```python
from build123d import *

# Parameters (mm, degrees)
BOSS_EXTRUDE1_DEPTH     = 6.35
F_1_4_CLEARANCE_HOLE1_D = 6.7564
FILLET1_R               = 2.54
SKETCH4_R               = 3.175
CUT_EXTRUDE1_DEPTH      = 7.3500001


with BuildPart() as part:
    # Sketch1 → Boss-Extrude1 (new body)
    with BuildSketch(Plane(origin=(0, 0, 0), x_dir=(1, 0, 0), z_dir=(0, 1, 0))):
        with BuildLine():
            ThreePointArc((34.041521739, -4.120545799), (22.86, 0), (34.041521739, 4.120545799))
            ThreePointArc((34.041521739, 4.120545799), (-34.29, 0), (34.041521739, -4.120545799))
        make_face()
    extrude(amount=BOSS_EXTRUDE1_DEPTH)

    # 1/4 Clearance Hole1 (through all)
    with Locations(Plane(origin=(0, 6.35, 0), x_dir=(1, 0, 0), z_dir=(0, 1, 0))):
        with Locations((0, 0)):
            Hole(F_1_4_CLEARANCE_HOLE1_D / 2)

    # Fillet1
    fillet1_edges = [part.edges().sort_by_distance(p)[0] for p in [
        (34.041521739, 3.175, 4.120545799),
        (34.041521739, 3.175, -4.120545799),
    ]]
    fillet(fillet1_edges, radius=FILLET1_R)

    # Sketch4 → Cut-Extrude1 (cut, through all)
    with BuildSketch(Plane(origin=(0, 6.35, 0), x_dir=(1, 0, 0), z_dir=(0, 1, 0))):
        with Locations((-14.86289651, -13.382612127)):
            Circle(SKETCH4_R)
    extrude(amount=-CUT_EXTRUDE1_DEPTH, mode=Mode.SUBTRACT)


solid = part.part
```
Design review of the part built by this model. Coordinates are the model's own, in mm. Give positions to 0.01 mm unless a question says otherwise; leave off trailing zeros. Order: outer loops, then holes, each group sorted by start corner. A loop starts at its lowest first (then second) coordinate and runs counter-clockwise, first axis right, second up. Notation, with made-up numbers: M 63.5,0 L 100.5,0 A26 ccw 100.5,21 Z; hole C 67.5,-19.75 d4. An arc over 180 degrees is marked long. One line per question, with ' | ' between items. Start each with the question number.
Q1. The part is to be moulded in two halves that separate along X. For faces 1 (the face through (-34.262, 3.131, -1.373)), 2 (the face through (22.86, 3.13, 0.15)), 3 (the face through (6, 6.35, 0)), say which applies: +X half, -X half, draft (parallel to the pull), parting line (faces both ways), or undercut.
Q2. We need section D-D (z = -17.5). Write out the cut boundary in (x, y), plus the area to 4 significant figures.
Q3. We need section A-A (x = 0). Write out the cut boundary in (y, z), plus the area to 3 significant figures.
Q4. For pin 1 Ø1 at (y, z) = (3, 26.5) entering from +X; pin 2 Ø7.5 at (x, z) = (-14.86, 13.38) entering from +Y; pin 3 Ø1 at (x, y) = (-24, 3) entering from -Z; pin 4 Ø1.5 at (y, z) = (2.5, 14) entering from -X, all flat-tipped, find the tip position at first contact; note any pin that passes through.
Q5. We need section B-B (z = 0). Write out the cut boundary in (x, y), plus the area to 3 significant figures.
Q6. We need section C-C (y = 1.25). State how many separate pieces and enclosed holes the cut face has, plus the area to 3 significant figures.
Q7. For L1, parallel to Z at x = 29.21, y = 1.5; L2, parallel to Z at x = 26, y = 1.25; L3, parallel to Z at x = 19.5, y = 5.75, list the stretches that pass through material, from the lowest coordinate up. Write a range as [from, to].
Returned:
1) face 1: parting line | face 2: undercut | face 3: draft
2) outline: M -29.49,0 L 29.49,0 L 29.49,6.35 L -29.49,6.35 Z | area: 374.5 mm2
3) outline: M 0,-34.29 L 6.35,-34.29 L 6.35,-3.38 L 0,-3.38 Z; M 0,3.38 L 6.35,3.38 L 6.35,34.29 L 0,34.29 Z | area: 393 mm2
4) pin 1: x = 22.36 | pin 2: y = 6.35 | pin 3: z = -24.97 | pin 4: x = -31.63
5) outline: M -34.29,0 L -3.38,0 L -3.38,6.35 L -34.29,6.35 Z; M 3.38,0 L 22.86,0 L 22.86,6.35 L 3.38,6.35 Z | area: 320 mm2
6) separate pieces: 1 | enclosed holes: 2 | area: 3,500 mm2
7) L1: [-17.96, -6.35], [6.35, 17.96] | L2: [-22.36, -5.48], [5.48, 22.36] | L3: [-28.21, 28.21]
